```python
from build123d import *

# Parameters (mm, degrees)
IZIM1_R                     = 2.5
Y_KSEKLIK_EKSTR_ZYON1_DEPTH = 19
SCALE1_SCALE                = 0.5


with BuildPart() as part:
    # Çizim1 → Yükseklik-Ekstrüzyon1 (new body)
    with BuildSketch(Plane.XY):
        Polygon((0.447956651, 4.923937404), (-4.544516536, 1.947612429), (-3.256622333, -3.720246726), (2.531813246, -4.246851352), (4.821368972, 1.095548245), align=None)
        Circle(IZIM1_R, mode=Mode.SUBTRACT)
    extrude(amount=Y_KSEKLIK_EKSTR_ZYON1_DEPTH)


with BuildPart() as part_1:
    # Scale1: scaled about (0, 0, 9.5)
    add(part.part.scale(SCALE1_SCALE).moved(Location((0, 0, 4.75))))


solid = part_1.part
```
Input: part model. Units: mm. Frame: model coordinates. Give positions to 0.01 mm unless a question says otherwise; leave off trailing zeros. Write each loop counter-clockwise with the first axis right and the second up, starting at its lowest first coordinate (ties: lowest second). Pieces come first, ordered by that corner, then holes. Notation, with made-up numbers: (-33, 22.25) - (-20, 22.25) arc R24 ccw to (-20, 53.25) - close; hole circle Ø6 at (79, 22.25). An arc over 180 degrees is marked (long way). Write item = value, one per line. Start each with the question number.
1) Cut plane D-D (y = 2.1). Return loops of the section in (x, z).
2) Cut plane B-B (y = 1.15). Return loops of the section in (x, z).
3) Cut plane A-A (x = -1.05). Return loops of the section in (y, z).
4) Pin query (flat end, axial travel): pin 1 (1.5 mm diameter, centred on x = -0.5, z = 10.5, fed in from -Y); pin 2 (1.5 mm diameter, centred on x = 0, y = 0, fed in from +Z); pin 3 (1.5 mm diameter, centred on y = 2, z = 6.5, fed in from +X); pin 4 (2 mm diameter, centred on x = 0, z = 9, fed in from -Y). Return the tip coordinate at first contact, or that it passes through.
5) Cut plane C-C (z = 8.5). Return loops of the section in (x, y).
6) Material intervals for L1, parallel to Y at x = 0, z = 9; L2, parallel to X at y = -0.8, z = 11.5; L3, parallel to Y at x = -0.55, z = 13.75, sorted ascending. Write a range as [from, to].
7) Draft query along X for faces 1 (the face through (-1, -1, 4.75)), 2 (the face through (-0.27, -1.22, 9.43)), 3 (the face through (-1.955, -0.423, 9.433)). Return one class per face: pulls with the +X half, pulls with the -X half, needs draft (parallel to the pull), parting line crosses it, or undercut.
Answers follow:
q1.outline = (-0.38, 4.75) - (0.64, 4.75) - (0.64, 14.25) - (-0.38, 14.25) - close
q2.outline = (-1.98, 4.75) - (-0.49, 4.75) - (-0.49, 14.25) - (-1.98, 14.25) - close; (0.49, 4.75) - (1.72, 4.75) - (1.72, 14.25) - (0.49, 14.25) - close
q3.outline = (-1.91, 4.75) - (-0.68, 4.75) - (-0.68, 14.25) - (-1.91, 14.25) - close; (0.68, 4.75) - (1.7, 4.75) - (1.7, 14.25) - (0.68, 14.25) - close
q4.pin_1 = -2.03
q4.pin_2 = through
q4.pin_3 = 1.61
q4.pin_4 = -2.1
q5.outline = (-2.27, 0.97) - (-1.63, -1.86) - (1.27, -2.12) - (2.41, 0.55) - (0.22, 2.46) - close; hole circle Ø2.5 at (0, 0)
q6.L1 = [-2.01, -1.25], [1.25, 2.33]
q6.L2 = [-1.87, -0.96], [0.96, 1.83]
q6.L3 = [-1.96, -1.12], [1.12, 2]
q7.face_1 = needs draft
q7.face_2 = undercut
q7.face_3 = pulls with the -X half
